Geometry check sheet. Reference: the model listing, model coordinates, mm. Give positions to 0.01 mm unless a question says otherwise; leave off trailing zeros. Loops run counter-clockwise (first coordinate to the right, second up) from the corner with the lowest first, then second, coordinate; pieces in that order, holes last. Notation, with made-up numbers: (11, 14) -> (48, 14) arc R8 ccw to (48, 28) -> close; hole circle Ø2 at (7, -31.5). An arc over 180 degrees is marked (long way). Write item = value, one per line. Start each with the question number.
```python
from build123d import *
from OCP.BRepFilletAPI import BRepFilletAPI_MakeFillet

# Parameters (mm, degrees)
FILLET1_R1 = 0.05
FILLET1_R2 = 0.15


with BuildPart() as part:
    # Sketch1 → Revolve1 (revolve)
    with BuildSketch(Plane(origin=(0, 0, 0), x_dir=(0, 0, -1), z_dir=(1, 0, 0)), mode=Mode.PRIVATE) as revolve1_sk:
        with BuildLine():
            Line((-10, 18.675), (-10, 17.825))
            Line((-10, 17.825), (9.450504516, 17.825))
            Line((9.450504516, 17.825), (10, 18.025))
            Line((10, 18.025), (10, 18.675))
            ThreePointArc((10, 18.675), (9.897487373, 18.922487373), (9.65, 19.025))
            Line((9.65, 19.025), (-9.65, 19.025))
            ThreePointArc((-9.65, 19.025), (-9.897487373, 18.922487373), (-10, 18.675))
        make_face()
    revolve(revolve1_sk.sketch.rotate(Axis((0, 0, 11.704423327), (0, 0, -1)), 90), axis=Axis((0, 0, 11.704423327), (0, 0, -1)))

    # Fillet1: one fillet with a radius per group of edges: ONE call of the kernel's fillet builder (fillet() takes one radius for all edges)
    fillet1_edges_1 = [part.edges().sort_by_distance(p)[0] for p in [
        (-18.025, 0, -10),
    ]]
    fillet1_edges_2 = [part.edges().sort_by_distance(p)[0] for p in [
        (-17.825, 0, -9.450504516),
    ]]
    fillet1 = BRepFilletAPI_MakeFillet(part.part.solid().wrapped)
    for e in fillet1_edges_1:
        fillet1.Add(FILLET1_R1, e.wrapped)
    for e in fillet1_edges_2:
        fillet1.Add(FILLET1_R2, e.wrapped)
    add(Compound.cast(fillet1.Shape()), mode=Mode.REPLACE)


solid = part.part
```
1) Draft check along Y on faces 1 (the cylindrical face through (-14.145, 10.846, 0.152)), 2 (the cylindrical face through (18.15, -5.71, 0.14)), 3 (the flat face through (7, 17, 10)). Enter one of: released by +Y, released by -Y, zero draft, split by the parting line, or undercut.
2) Section check A-A (z = 1.5). Enter the section's corners in (x, y) (3 decimals), plus the area to 3 significant figures.
3) Thickness scan on line 1 (Y direction, x = 0, z = 4.5) (3 decimals); line 2 (Y direction, x = 13, z = -5.5); line 3 (X direction, y = -6, z = -5.5). Record the ranges inside material, lowest first.
4) Depth check by flat-ended pin: pin 1 Ø5 at (y, z) = (-14, 0.5) entering from -X; pin 2 Ø2 at (x, z) = (-0.5, -3.5) entering from -Y (3 decimals); pin 3 Ø2 at (y, z) = (-4, -2) entering from -X. Enter the tip coordinate at first touch or a pass-through.
Check result:
q1.face_1 = undercut
q1.face_2 = split by the parting line
q1.face_3 = zero draft
q2.outline = circle Ø38.05 at (0, 0); hole circle Ø35.65 at (0, 0)
q2.area = 139 mm2
q3.line_1 = -19.025 to -17.825, 17.825 to 19.025
q3.line_2 = -13.89 to -12.2, 12.2 to 13.89
q3.line_3 = -18.05 to -16.78, 16.78 to 18.05
q4.pin_1 = -15.16
q4.pin_2 = -19.025
q4.pin_3 = -18.79
